```python
from build123d import *

# Parameters (mm, degrees)
F1_W      = 75
F1_H      = 98
F2_DEPTH  = 1.5
F3_W      = 75
F3_H      = 98
F4_DEPTH  = 6.7
F5_W      = 9.7
F5_H      = 56
F5_H_2    = 11.5
F5_H_3    = 23
F6_DEPTH  = 25
F7_R      = 1.6
F8_R      = 1.6
F9_DEPTH  = 25
F10_W     = 2
F10_H     = 54.75
F11_DEPTH = 5
F12_R     = 2


with BuildPart() as f2:
    # F1 (on Top) → F2 (new body)
    with BuildSketch(Plane.XY):
        with Locations((-2, -1.5)):
            Rectangle(F1_W, F1_H)
    extrude(amount=F2_DEPTH)

    # F3 (on face) → F4 (join)
    with BuildSketch(Plane(origin=(0, 0, 0), x_dir=(1, 0, 0), z_dir=(0, 0, -1))):
        with Locations((-2, 1.5)):
            Rectangle(F3_W, F3_H)
        Polygon((25.5, -37.5), (25.5, -45.5), (-29.5, -45.5), (-29.5, -37.5), (-37.5, -37.5), (-37.5, 40.5), (-29.5, 40.5), (-29.5, 48.5), (25.5, 48.5), (25.5, 40.5), (33.5, 40.5), (33.5, -37.5), align=None, mode=Mode.SUBTRACT)
    extrude(amount=F4_DEPTH)

    # F5 (on face) → F6 (cut)
    with BuildSketch(Plane(origin=(0, 0, -6.7), x_dir=(1, 0, 0), z_dir=(0, 0, -1))):
        with Locations((-34.65, -8.25)):
            Rectangle(F5_W, F5_H)
        with Locations((-34.65, 34.5)):
            Rectangle(F5_W, F5_H_2)
        with Locations((30.65, 28.75)):
            Rectangle(F5_W, F5_H_3)
    extrude(amount=-F6_DEPTH, mode=Mode.SUBTRACT)

    # F7 (on face) + F8 (on face) → F9 (cut)
    with BuildSketch(Plane(origin=(0, 0, -6.7), x_dir=(1, 0, 0), z_dir=(0, 0, -1))):
        with Locations((29, -41)):
            Circle(F7_R)
        with Locations((-33, -41)):
            Circle(F7_R)
    with BuildSketch(Plane(origin=(0, 0, -6.7), x_dir=(1, 0, 0), z_dir=(0, 0, -1))):
        with Locations((-33, 44)):
            Circle(F8_R)
        with Locations((29, 44)):
            Circle(F8_R)
    extrude(amount=-F9_DEPTH, mode=Mode.SUBTRACT)

    # F10 (on face) → F11 (cut)
    with BuildSketch(Plane(origin=(0, 0, -6.7), x_dir=(1, 0, 0), z_dir=(0, 0, -1))):
        with Locations((34.5, -10.125)):
            Rectangle(F10_W, F10_H)
    extrude(amount=-F11_DEPTH, mode=Mode.SUBTRACT)

    # F12
    f12_edges = [f2.edges().sort_by_distance(p)[0] for p in [
        (-39.5, 47.5, -2.6),
        (35.5, 47.5, -2.6),
        (-39.5, -50.5, -2.6),
        (35.5, -50.5, -2.6),
    ]]
    fillet(f12_edges, radius=F12_R)


solid = f2.part
```
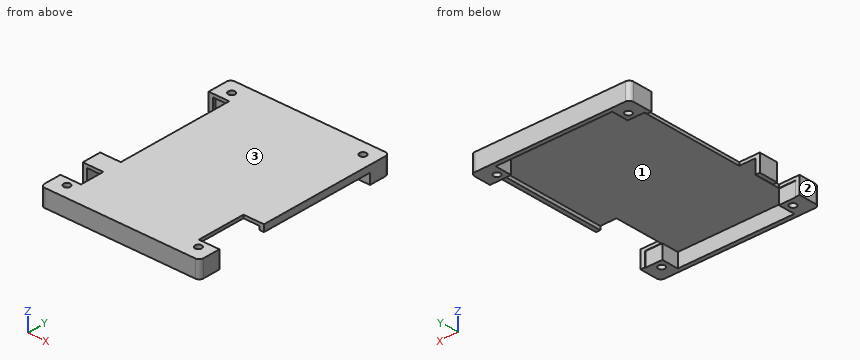
Check sheet for the modelled part. Datum: model origin and axes. Units: mm. Face numbers are marked on the shaded views. Coordinates: 2 decimals unless noted, no trailing zeros. Write each loop counter-clockwise with the first axis right and the second up, starting at its lowest first coordinate (ties: lowest second). Pieces come first, ordered by that corner, then holes. Notation, with made-up numbers: (-38.75, 89.5) - (-29.75, 89.5) arc R26 ccw to (-29.75, 103.5) - close; hole circle Ø7 at (4.25, -34.5). An arc over 180 degrees is marked (long way). One line per question, with ' | ' between items.
Item 1: Sectioned sample at A-A on y = 41. Record the boundary of the cut face in (x, z), plus the area to 3 significant figures.
Determined:
outline: (-39.5, -6.7) - (-34.6, -6.7) - (-34.6, 1.5) - (-39.5, 1.5) - close; (-31.4, -6.7) - (-29.5, -6.7) - (-29.5, 0) - (25.5, 0) - (25.5, -6.7) - (27.4, -6.7) - (27.4, 1.5) - (-31.4, 1.5) - close; (30.6, -6.7) - (35.5, -6.7) - (35.5, 1.5) - (30.6, 1.5) - close | area: 194 mm2
Item 2: Sectioned sample at C-C on x = 29. Record the boundary of the cut face in (y, z), plus the area to 3 significant figures.
Determined:
outline: (-50.5, -6.7) - (-45.6, -6.7) - (-45.6, 1.5) - (-50.5, 1.5) - close; (-42.4, -6.7) - (-40.5, -6.7) - (-40.5, 0) - (-40.25, 0) - (-40.25, 1.5) - (-42.4, 1.5) - close; (-17.25, 0) - (37.5, 0) - (37.5, -6.7) - (39.4, -6.7) - (39.4, 1.5) - (-17.25, 1.5) - close; (42.6, -6.7) - (47.5, -6.7) - (47.5, 1.5) - (42.6, 1.5) - close | area: 194 mm2
Item 3: Sectioned sample at D-D on x = -33. Record the boundary of the cut face in (y, z).
Determined:
outline: (-50.5, -6.7) - (-45.6, -6.7) - (-45.6, 1.5) - (-50.5, 1.5) - close; (-42.4, -6.7) - (-40.5, -6.7) - (-40.5, 0) - (-40.25, 0) - (-40.25, 1.5) - (-42.4, 1.5) - close; (-28.75, 0) - (-19.75, 0) - (-19.75, 1.5) - (-28.75, 1.5) - close; (36.25, 0) - (37.5, 0) - (37.5, -6.7) - (39.4, -6.7) - (39.4, 1.5) - (36.25, 1.5) - close; (42.6, -6.7) - (47.5, -6.7) - (47.5, 1.5) - (42.6, 1.5) - close
Item 4: Gauge pin test, flat ends, axial feed: P1, Ø1.2, axis at y = -31.5, z = 1, coming from the +X side; P2, Ø4, axis at x = -10, y = -18, coming from the -Z side; P3, Ø3.5, axis at x = 29, y = 41, coming from the -Z side; P4, Ø1.4, axis at y = 19, z = -1, coming from the -X side. Record the tip position at first contact, or that the pin passes through.
Determined:
P1: stops at x = 25.8 | P2: stops at z = 0 | P3: stops at z = -6.7 | P4: stops at x = 33.5
Item 5: Mould release check, pull along X, two halves, no side actions. Record for the marked faces 1, 2 and 3: pulls with the +X half, pulls with the -X half, needs draft (parallel to the pull), parting line crosses it, or undercut.
Determined:
face 1: undercut | face 2: pulls with the -X half | face 3: needs draft
Item 6: Thickness scan on line 1 (Y direction, x = -33, z = -2.75); line 2 (X direction, y = 41, z = -3); line 3 (Y direction, x = -20, z = -4.5). Record the ranges inside material, lowest first. Write a range as [from, to].
Determined:
line 1: y = [-50.5, -45.6], [-42.4, -40.5], [37.5, 39.4], [42.6, 47.5] | line 2: x = [-39.5, -34.6], [-31.4, -29.5], [25.5, 27.4], [30.6, 35.5] | line 3: y = [-50.5, -48.5], [45.5, 47.5]
Item 7: Sectioned sample at B-B on z = -4.5. Give the number of separate pieces and of enclosed holes in the cut face, plus the area to 3 significant figures.
Determined:
separate pieces: 3 | enclosed holes: 4 | area: 606 mm2
